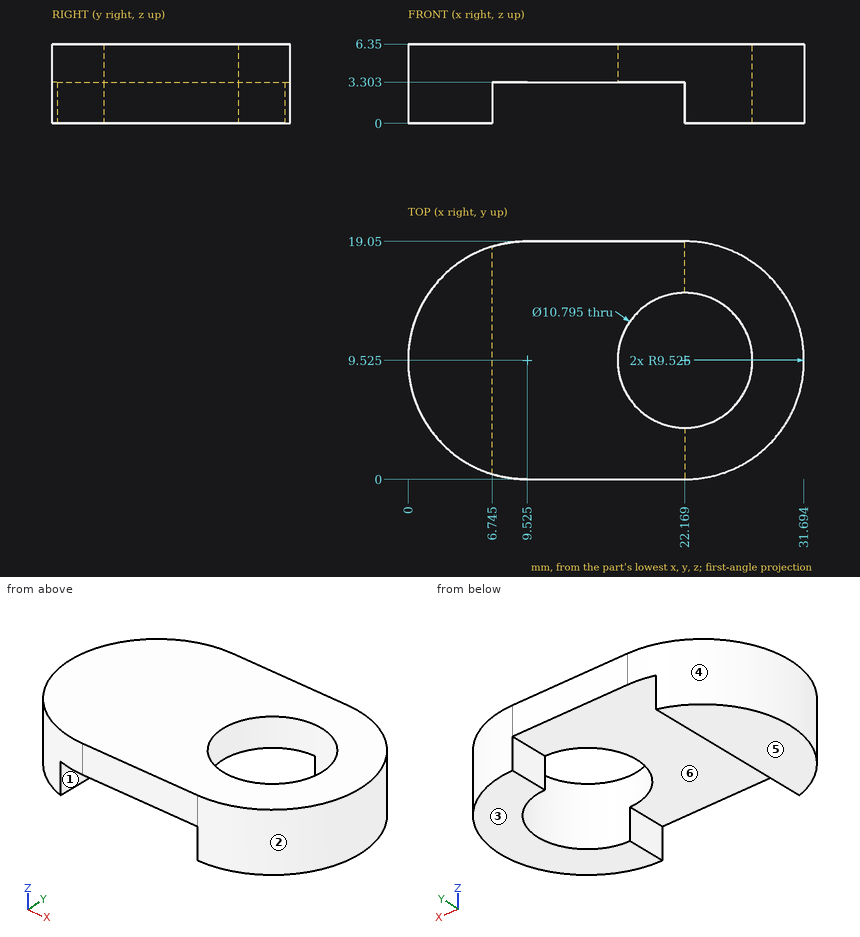
Here's the drawing with two shaded views (mm, measured from the low corner). I have some questions. A direction names the side the tool comes from. Give positions to 0.01 mm unless a question says otherwise; leave off trailing zeros. Use one line per item in the form item = value.
1) If I drill on L1, parallel to X at y = 9.5, z = 0.75 (1 decimal); L2, parallel to Z at x = 18, y = 13; L3, parallel to X at y = 4.75, z = 3.75 (1 decimal), over which ranges is the centre line in solid material (lowest first)? Write a range as [from, to].
Verdict:
L1 = [0, 6.7], [27.6, 31.7]
L2 = [3.3, 6.35]
L3 = [1.3, 19.7], [24.7, 30.4]
2) I'm going to push flat-ended pins straight in: pin 1 (1.5 mm diameter, centred on y = 7.5, z = 4.5, fed in from +X); pin 2 (2.5 mm diameter, centred on y = 2.5, z = 1, fed in from -X); pin 3 (3.5 mm diameter, centred on y = 11.5, z = 2, fed in from +X); pin 4 (1 mm diameter, centred on x = 27, y = 10, fed in from -Z). Where does each tip first touch, or does it pass through?
Verdict:
pin_1 = 31.61
pin_2 = 1.95
pin_3 = 31.69
pin_4 = through
3) On a 3-axis mill with a long thin cutter (end or side, diameter ignored), from which of +Z, -Z, +X, -X, +Y, -Y can I reach the whole of each face in a straight line? I mean the marked faces 5 and 6. Say none if no direction works.
Verdict:
face_5 = -Z, +X, -X, +Y, -Y
face_6 = -Z, +Y, -Y
4) We'd pull the mould along X, two halves only. Please class the marked faces 1, 2, 3 and 4: +X half, -X half, draft (parallel to the pull), parting line (faces both ways), or undercut.
Verdict:
face_1 = undercut
face_2 = +X half
face_3 = draft
face_4 = -X half
